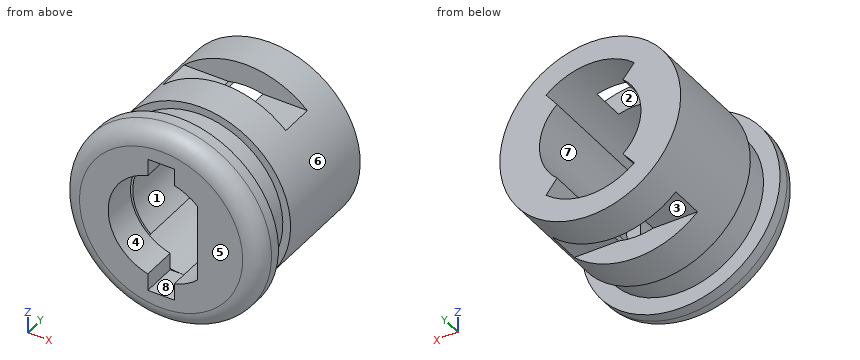
```python
from build123d import *

# Parameters (mm, degrees)
CROQUIS1_R                 = 4.5
SALIENTE_EXTRUIR1_DEPTH    = 1.3
CROQUIS2_R                 = 3.75
SALIENTE_EXTRUIR2_DEPTH    = 1.5
CROQUIS3_R                 = 4.1
SALIENTE_EXTRUIR3_DEPTH    = 5
CORTAR_EXTRUIR3_DEPTH      = 6.2
CORTAR_EXTRUIR4_DEPTH      = 1.8
REDONDEO1_R                = 0.8
CORTAR_EXTRUIR5_DEPTH      = 11.066777041
CORTAR_EXTRUIR5_DEPTH_BACK = 11.066777041
CROQUIS8_W                 = 1.1
CROQUIS8_H                 = 1.55


with BuildPart() as part:
    # Croquis1 → Saliente-Extruir1 (new body)
    with BuildSketch(Plane(origin=(0, 0, 0), x_dir=(1, 0, 0), z_dir=(0, 1, 0))):
        with Locations(Location((0, 0, 0), (0, 0, 270))):
            Circle(CROQUIS1_R)
    extrude(amount=SALIENTE_EXTRUIR1_DEPTH)

    # Croquis2 → Saliente-Extruir2 (add)
    with BuildSketch(Plane(origin=(0, 1.3, 0), x_dir=(1, 0, 0), z_dir=(0, 1, 0))):
        with Locations(Location((0, 0, 0), (0, 0, 270))):
            Circle(CROQUIS2_R)
    extrude(amount=SALIENTE_EXTRUIR2_DEPTH)

    # Croquis3 → Saliente-Extruir3 (add)
    with BuildSketch(Plane(origin=(0, 2.8, 0), x_dir=(1, 0, 0), z_dir=(0, 1, 0))):
        with Locations(Location((0, 0, 0), (0, 0, 270))):
            Circle(CROQUIS3_R)
    extrude(amount=SALIENTE_EXTRUIR3_DEPTH)

    # Croquis4 → Cortar-Extruir3 (cut)
    with BuildSketch(Plane(origin=(0, 7.8, 0), x_dir=(1, 0, 0), z_dir=(0, 1, 0))):
        with BuildLine():
            Line((-2, 2.368543856), (-1.483870968, 1.757306732))
            ThreePointArc((-1.483870968, 1.757306732), (-2.3, 0), (-1.483870968, -1.757306732))
            Line((-1.483870968, -1.757306732), (-2, -2.368543856))
            ThreePointArc((-2, -2.368543856), (0, -3.1), (2, -2.368543856))
            Line((2, -2.368543856), (1.503663664, -1.740400984))
            ThreePointArc((1.503663664, -1.740400984), (2.3, 0), (1.503663664, 1.740400984))
            Line((1.503663664, 1.740400984), (2, 2.368543856))
            ThreePointArc((2, 2.368543856), (0, 3.1), (-2, 2.368543856))
        make_face()
    extrude(amount=-CORTAR_EXTRUIR3_DEPTH, mode=Mode.SUBTRACT)

    # Croquis7 → Cortar-Extruir4 (cut)
    with BuildSketch(Plane(origin=(0, 1.6, 0), x_dir=(1, 0, 0), z_dir=(0, 1, 0))):
        with BuildLine():
            Line((1.642406771, 1.75), (1.642406771, -1.75))
            ThreePointArc((1.642406771, -1.75), (1.157326995, -2.102520922), (0.6, -2.323790008))
            Line((0.6, -2.323790008), (0.6, -3.1))
            Line((0.6, -3.1), (-0.6, -3.1))
            Line((-0.6, -3.1), (-0.6, -2.323790008))
            ThreePointArc((-0.6, -2.323790008), (-2.4, 0), (-0.6, 2.323790008))
            Line((-0.6, 2.323790008), (-0.6, 3.1))
            Line((-0.6, 3.1), (0.6, 3.1))
            Line((0.6, 3.1), (0.6, 2.323790008))
            ThreePointArc((0.6, 2.323790008), (1.157326995, 2.102520922), (1.642406771, 1.75))
        make_face()
    extrude(amount=-CORTAR_EXTRUIR4_DEPTH, mode=Mode.SUBTRACT)

    # Redondeo1
    redondeo1_edges = [part.edges().sort_by_distance(p)[0] for p in [
        (0, 0, -4.5),
    ]]
    fillet(redondeo1_edges, radius=REDONDEO1_R)

    # Croquis8 → Cortar-Extruir5 (cut, two sides: drawn at the far end of the back side and taken through both)
    with BuildSketch(Plane(origin=(0, 0, 0), x_dir=(0, 0, -1), z_dir=(1, 0, 0)).offset(-CORTAR_EXTRUIR5_DEPTH_BACK)):
        with Locations((-3.55, 5.3)):
            Rectangle(CROQUIS8_W, CROQUIS8_H)
        with Locations((3.55, 5.3)):
            Rectangle(CROQUIS8_W, CROQUIS8_H)
    extrude(amount=CORTAR_EXTRUIR5_DEPTH + CORTAR_EXTRUIR5_DEPTH_BACK, mode=Mode.SUBTRACT)


solid = part.part
```
Build history of the part. All positions in model axes, mm. Face numbers are marked on the shaded views. A direction names the side the tool comes from. Round coordinates to 2 decimals unless told otherwise and drop trailing zeros. Write each loop counter-clockwise with the first axis right and the second up, starting at its lowest first coordinate (ties: lowest second). Pieces come first, ordered by that corner, then holes. Notation, with made-up numbers: (77.25, 37.5) - (108.25, 37.5) arc R27 ccw to (108.25, 76.5) - close; hole circle Ø4 at (87, 56.25). An arc over 180 degrees is marked (long way). Write each question's results on one line, items separated by ' | '. Start each with the question number.
Item 1: Wall check: L1, parallel to Y at x = -1.25, z = 3.5 (3 decimals); L2, parallel to X at y = 2.5, z = 2.5; L3, parallel to X at y = 0.75, z = -0.75. Give the ranges that are in metal, low to high. Write a range as [from, to].
Item 2: Mould opens along X. For the marked faces 5, 6, 7 and 8 say: pulls with the +X half, pulls with the -X half, needs draft (parallel to the pull), parting line crosses it, or undercut.
Item 3: Saw through at A-A (z = 0). Write the cut outline in (x, y), and give its area (3 significant figures).
Item 4: Saw through at B-B (y = 4). Write the cut outline in (x, z).
Item 5: Drop flat-ended pins along their axis: P1, Ø0.6, axis at x = -1.5, z = -2.5, coming from the +Y side; P2, Ø2, axis at y = 4.5, z = -3, coming from the -X side; P3, Ø0.5, axis at x = -1.5, y = 5, coming from the -Z side; P4, Ø1.7, axis at x = 2, y = 5, coming from the +Z side. Give the stop position or say it passes through.
Item 6: Saw through at C-C (y = 2.5). Write the cut outline in (x, z), and give its area (3 significant figures).
Item 7: Which spindle directions (+Z, -Z, +X, -X, +Y, -Y) get a long thin tool onto all of the face, cutting with end or side? Do the marked faces 1, 2, 3 and 4. Say none if no direction does.
Results are:
1) L1: y = [0, 4.525], [6.075, 7.8] | L2: x = [-2.8, -1.83], [1.83, 2.8] | L3: x = [-4.44, -2.28], [1.64, 4.44]
2) face 5: needs draft | face 6: parting line crosses it | face 7: undercut | face 8: undercut
3) outline: (-4.5, 0.8) arc R0.8 ccw to (-3.7, 0) - (-2.4, 0) - (-2.4, 1.6) - (-2.3, 1.6) - (-2.3, 7.8) - (-4.1, 7.8) - (-4.1, 2.8) - (-3.75, 2.8) - (-3.75, 1.3) - (-4.5, 1.3) - close; (1.64, 0) - (3.7, 0) arc R0.8 ccw to (4.5, 0.8) - (4.5, 1.3) - (3.75, 1.3) - (3.75, 2.8) - (4.1, 2.8) - (4.1, 7.8) - (2.3, 7.8) - (2.3, 1.6) - (1.64, 1.6) - close | area: 28.7 mm²
4) outline: circle Ø8.2 at (0, 0); hole (-2, -2.37) arc R3.1 ccw to (2, -2.37) - (1.5, -1.74) arc R2.3 ccw to (1.5, 1.74) - (2, 2.37) arc R3.1 ccw to (-2, 2.37) - (-1.48, 1.76) arc R2.3 ccw to (-1.48, -1.76) - close
5) P1: stops at y = 7.8 | P2: stops at x = -3.58 | P3: stops at z = -3 | P4: stops at z = 3.89
6) outline: circle Ø7.5 at (0, 0); hole (-2, -2.37) arc R3.1 ccw to (2, -2.37) - (1.5, -1.74) arc R2.3 ccw to (1.5, 1.74) - (2, 2.37) arc R3.1 ccw to (-2, 2.37) - (-1.48, 1.76) arc R2.3 ccw to (-1.48, -1.76) - close | area: 21.5 mm²
7) face 1: +Y, -Y | face 2: +Z, +X, -X | face 3: -Z, +X, -X | face 4: -Y
